from build123d import *

# Parameters (mm, degrees)
BOSS_EXTRUDE1_DEPTH     = 35
CUT_EXTRUDE1_DEPTH      = 165.23458831805192
CUT_EXTRUDE1_DEPTH_BACK = 165.23458831805192
CUT_EXTRUDE2_START      = 35
CUT_EXTRUDE2_DEPTH      = 10.61
SKETCH5_R               = 1.600000000000005
SKETCH5_R_2             = 1.6000000000000056
CUT_EXTRUDE3_DEPTH      = 165.23458831805192
SKETCH5_3_R             = 3.0000000000000004
SKETCH5_3_R_2           = 3.0000000000000013
CUT_EXTRUDE4_DEPTH      = 21
SKETCH8_R               = 1.600000000000005
SKETCH8_R_2             = 1.6000000000000056
CUT_EXTRUDE5_DEPTH      = 165.23458831805192
SKETCH8_3_R             = 3.000000000000008
CUT_EXTRUDE6_DEPTH      = 25
CUT_EXTRUDE7_REACH      = 166.235
SKETCH7_R               = 4.1
SKETCH7_R_2             = 4.099999999999986
SKETCH7_3_R             = 11
SKETCH7_3_R_2           = 10.999999999999993
CUT_EXTRUDE8_DEPTH      = 7.1
CUT_EXTRUDE9_DEPTH      = 21
CUT_EXTRUDE11_START     = 24.39
SKETCH11_R              = 11.6
CUT_EXTRUDE11_DEPTH     = 189.6245883180519
FILLET3_R               = 9
FILLET4_R               = 9


with BuildPart() as part:
    # Sketch1 → Boss-Extrude1 (new body)
    with BuildSketch(Plane(origin=(0, 0, 0), x_dir=(0, 0, -1), z_dir=(1, 0, 0))):
        with BuildLine():
            ThreePointArc((-3.4331525583588727, 27.788729073331762), (-20.97770568525129, 18.545507924642443), (-28, 3.43e-15))
            Line((-28, 0), (28, 0))
            ThreePointArc((28, 0), (18.545507924642447, 20.977705685251287), (-3.4331525583588727, 27.788729073331762))
        make_face()
        with BuildLine():
            Line((28, 0), (-28, 0))
            ThreePointArc((-28, 3.43e-15), (-20.977705685251298, -18.545507924642436), (-3.433152558358892, -27.78872907333176))
            ThreePointArc((-3.433152558358892, -27.78872907333176), (18.545507924642436, -20.977705685251298), (28, -6.86e-15))
        make_face()
        with BuildLine():
            ThreePointArc((-126.56684744164114, 27.788729073331766), (-109.02229431474872, 18.54550792464245), (-102, 0))
            Line((-102, 0), (-28, 0))
            ThreePointArc((-28, 3.43e-15), (-20.97770568525129, 18.545507924642443), (-3.4331525583588727, 27.788729073331762))
            ThreePointArc((-3.433152558358863, 27.788729073331695), (-65, 23.999999999999602), (-126.56684744164116, 27.788729073331638))
        make_face()
        with BuildLine():
            Line((-28, 0), (-102, 0))
            ThreePointArc((-102, -6.86e-15), (-109.0222943147487, -18.545507924642447), (-126.56684744164114, -27.788729073331766))
            ThreePointArc((-126.56684744164116, -27.788729073331638), (-65, -23.999999999999602), (-3.433152558358863, -27.788729073331695))
            ThreePointArc((-3.433152558358892, -27.78872907333176), (-20.977705685251298, -18.545507924642436), (-28, 3.43e-15))
        make_face()
        with BuildLine():
            ThreePointArc((-126.56684744164114, 27.788729073331766), (-148.54550792464244, 20.977705685251287), (-158, 3.43e-15))
            Line((-158, 0), (-102, 0))
            ThreePointArc((-102, 0), (-109.02229431474872, 18.54550792464245), (-126.56684744164114, 27.788729073331766))
        make_face()
        with BuildLine():
            Line((-102, 0), (-158, 0))
            ThreePointArc((-158, 3.43e-15), (-148.54550792464244, -20.97770568525128), (-126.56684744164114, -27.788729073331766))
            ThreePointArc((-126.56684744164114, -27.788729073331766), (-109.0222943147487, -18.545507924642447), (-102, -6.86e-15))
        make_face()
    extrude(amount=BOSS_EXTRUDE1_DEPTH)

    # Sketch4 → Cut-Extrude1 (cut, two sides: drawn at the far end of the back side and taken through both)
    with BuildSketch(Plane(origin=(0, 0, 0), x_dir=(1, 0, 0), z_dir=(0, 1, 0)).offset(-CUT_EXTRUDE1_DEPTH_BACK)):
        Polygon((8.999999999999998, 27.999999999999996), (61, 27.999999999999996), (61, -28.000000000000004), (9.000000000000005, -28.000000000000004), align=None)
        Polygon((60.999999999999986, -157.99999999999997), (60.99999999999993, -101.99999999999999), (8.999999999999956, -101.99999999999999), (8.99999999999997, -157.99999999999997), align=None)
    extrude(amount=CUT_EXTRUDE1_DEPTH + CUT_EXTRUDE1_DEPTH_BACK, mode=Mode.SUBTRACT)

    # Sketch6 → Cut-Extrude2 (cut)
    with BuildSketch(Plane(origin=(0, 0, 0), x_dir=(0, 0, -1), z_dir=(1, 0, 0)).offset(CUT_EXTRUDE2_START)):
        Polygon((-27.624999999999996, -21.1), (-69.825, -21.100000000000005), (-69.825, 21.099999999999994), (-27.624999999999996, 21.1), align=None)
    extrude(amount=-CUT_EXTRUDE2_DEPTH, mode=Mode.SUBTRACT)

    # Sketch5 → Cut-Extrude3 (cut, through all)
    with BuildSketch(Plane(origin=(0, 0, 0), x_dir=(0, 0, -1), z_dir=(1, 0, 0))):
        with Locations(Location((-33.225, -15.5, 0), (0, 0, 180))):
            Circle(SKETCH5_R)
        with Locations(Location((-33.225, 15.5, 0), (0, 0, 180))):
            Circle(SKETCH5_R)
        with Locations(Location((-64.22500000000001, -15.500000000000004, 0), (0, 0, 180))):
            Circle(SKETCH5_R)
        with Locations(Location((-64.22500000000001, 15.499999999999995, 0), (0, 0, 180))):
            Circle(SKETCH5_R_2)
    extrude(amount=CUT_EXTRUDE3_DEPTH, mode=Mode.SUBTRACT)

    # Sketch5<3> → Cut-Extrude4 (cut)
    with BuildSketch(Plane(origin=(0, 0, 0), x_dir=(0, 0, -1), z_dir=(1, 0, 0))):
        with Locations(Location((-33.225, -15.5, 0), (0, 0, 180))):
            Circle(SKETCH5_3_R)
        with Locations(Location((-33.225, 15.5, 0), (0, 0, 180))):
            Circle(SKETCH5_3_R)
        with Locations(Location((-64.22500000000001, -15.500000000000004, 0), (0, 0, 180))):
            Circle(SKETCH5_3_R_2)
        with Locations(Location((-64.22500000000001, 15.499999999999995, 0), (0, 0, 180))):
            Circle(SKETCH5_3_R_2)
    extrude(amount=CUT_EXTRUDE4_DEPTH, mode=Mode.SUBTRACT)

    # Sketch8 → Cut-Extrude5 (cut, through all)
    with BuildSketch(Plane(origin=(0, 0, 0), x_dir=(0, 0, -1), z_dir=(1, 0, 0))):
        with Locations((-94, -15.500000000000012)):
            Circle(SKETCH8_R)
        with Locations((-94, 15.499999999999988)):
            Circle(SKETCH8_R_2)
    extrude(amount=CUT_EXTRUDE5_DEPTH, mode=Mode.SUBTRACT)

    # Sketch8<3> → Cut-Extrude6 (cut)
    with BuildSketch(Plane(origin=(0, 0, 0), x_dir=(0, 0, -1), z_dir=(1, 0, 0))):
        with Locations((-94, -15.500000000000012)):
            Circle(SKETCH8_3_R)
        with Locations((-94, 15.499999999999988)):
            Circle(SKETCH8_3_R)
    extrude(amount=CUT_EXTRUDE6_DEPTH, mode=Mode.SUBTRACT)

    # Sketch7 → Cut-Extrude7 (cut, up to next)
    with BuildSketch(Plane(origin=(0, 0, 0), x_dir=(0, 0, -1), z_dir=(1, 0, 0)), mode=Mode.PRIVATE) as cut_extrude7_sk1:
        with Locations(Location((0, 0, 0), (0, 0, 180))):
            Circle(SKETCH7_R)
    cut_extrude7_tool1 = extrude(cut_extrude7_sk1.sketch, amount=CUT_EXTRUDE7_REACH, mode=Mode.PRIVATE) & part.part
    # Sketch7 → Cut-Extrude7 (cut, up to next)
    with BuildSketch(Plane(origin=(0, 0, 0), x_dir=(0, 0, -1), z_dir=(1, 0, 0)), mode=Mode.PRIVATE) as cut_extrude7_sk2:
        with Locations(Location((-130, 0, 0), (0, 0, 180))):
            Circle(SKETCH7_R_2)
    cut_extrude7_tool2 = extrude(cut_extrude7_sk2.sketch, amount=CUT_EXTRUDE7_REACH, mode=Mode.PRIVATE) & part.part
    add(cut_extrude7_tool1.solids().sort_by_distance((0, 0, 0))[0], mode=Mode.SUBTRACT)
    add(cut_extrude7_tool2.solids().sort_by_distance((0, 0, 130))[0], mode=Mode.SUBTRACT)

    # Sketch7<3> → Cut-Extrude8 (cut)
    with BuildSketch(Plane(origin=(0, 0, 0), x_dir=(0, 0, -1), z_dir=(1, 0, 0))):
        Circle(SKETCH7_3_R)
        with Locations((-130, 0)):
            Circle(SKETCH7_3_R_2)
    extrude(amount=CUT_EXTRUDE8_DEPTH, mode=Mode.SUBTRACT)

    # Sketch9 → Cut-Extrude9 (cut)
    with BuildSketch(Plane(origin=(0, 0, 0), x_dir=(0, 0, -1), z_dir=(1, 0, 0))):
        with BuildLine():
            Line((-52.942405411719506, -6.7980505730098315), (-34.806527029394815, -18.04926896487869))
            ThreePointArc((-34.80652702939481, -18.049268964878678), (-34.68366701337481, -12.878494603459266), (-30.22500000000001, -15.5))
            Line((-30.225000000000005, -15.5), (-30.225000000000005, 15.5))
            ThreePointArc((-30.225, 15.5), (-34.68366701337481, 12.878494603459261), (-34.806527029394815, 18.04926896487868))
            Line((-34.806527029394815, 18.04926896487869), (-52.942405411719506, 6.7980505730098315))
            ThreePointArc((-52.9424054117195, 6.7980505730098155), (-56.725, 9.8e-16), (-52.9424054117195, -6.798050573009815))
        make_face()
    extrude(amount=CUT_EXTRUDE9_DEPTH, mode=Mode.SUBTRACT)

    # Sketch11 → Cut-Extrude11 (cut, through all)
    with BuildSketch(Plane(origin=(0, 0, 0), x_dir=(0, 0, -1), z_dir=(1, 0, 0)).offset(CUT_EXTRUDE11_START)):
        with Locations(Location((-48.725, 0, 0), (0, 0, 75.417643506))):
            Circle(SKETCH11_R)
    extrude(amount=-CUT_EXTRUDE11_DEPTH, mode=Mode.SUBTRACT)

    # Fillet3
    # the kernel refuses this fillet: 9 mm, written as the material it takes off along each edge
    with BuildSketch(Plane(origin=(0, -7.11e-15, 130), x_dir=(0, 0.9924546097618487, -0.12261259136995861), z_dir=(0, -0.12261259136995861, -0.9924546097618487))) as fillet3_piece_1:
        with BuildLine():
            CenterArc((28 - FILLET3_R, FILLET3_R), FILLET3_R, 270, 89.99999999999999)
            Line((28, FILLET3_R), (28, 0))
            Line((28, 0), (28 - FILLET3_R, 0))
        make_face()
    revolve(axis=Axis((0, -7.11e-15, 130), (1, 0, 0)), revolution_arc=194.0858135076888, mode=Mode.SUBTRACT)
    with BuildSketch(Plane(origin=(0, -526.1249999999588, 65.00000000000026), x_dir=(0, 0.9924546097618475, 0.12261259136996942), z_dir=(0, -0.12261259136996942, 0.9924546097618475))) as fillet3_piece_2:
        with BuildLine():
            CenterArc((502.1249999999593 + FILLET3_R, -FILLET3_R), FILLET3_R, 90, 90)
            Line((502.1249999999593 + FILLET3_R, 1.78e-15), (502.1249999999593, 0))
            Line((502.1249999999593, 0), (502.1249999999593, -FILLET3_R))
        make_face()
    revolve(axis=Axis((0, -526.1249999999588, 65.00000000000026), (-1, 0, 0)), revolution_arc=14.085813507690109, mode=Mode.SUBTRACT)
    with BuildSketch(Plane(origin=(0, 1.78e-15, -1.78e-15), x_dir=(0, -0.9924546097618486, 0.12261259136995943), z_dir=(0, 0.12261259136995943, 0.9924546097618486))) as fillet3_piece_3:
        with BuildLine():
            CenterArc((27.999999999999993 - FILLET3_R, FILLET3_R), FILLET3_R, 270, 89.99999999999999)
            Line((27.999999999999993, FILLET3_R), (27.999999999999993, 0))
            Line((27.999999999999993, 0), (27.999999999999993 - FILLET3_R, 0))
        make_face()
    revolve(axis=Axis((0, 1.78e-15, -1.78e-15), (1, 0, 0)), revolution_arc=194.0858135076889, mode=Mode.SUBTRACT)
    with BuildSketch(Plane(origin=(0, 526.1249999999663, 65.00000000000024), x_dir=(0, -0.9924546097618476, -0.12261259136996856), z_dir=(0, 0.12261259136996856, -0.9924546097618476))) as fillet3_piece_4:
        with BuildLine():
            CenterArc((502.1249999999667 + FILLET3_R, -FILLET3_R), FILLET3_R, 90, 90)
            Line((502.1249999999667 + FILLET3_R, 1.78e-15), (502.1249999999667, 0))
            Line((502.1249999999667, 0), (502.1249999999667, -FILLET3_R))
        make_face()
    revolve(axis=Axis((0, 526.1249999999663, 65.00000000000024), (-1, 0, 0)), revolution_arc=14.085813507689899, mode=Mode.SUBTRACT)

    # Fillet4
    fillet4_edges = [part.edges().sort_by_distance(p)[0] for p in [
        (22.000000000000004, -25.365061880944552, 28),
        (21.99999999999998, -25.365061880944495, 101.99999999999999),
        (21.99999999999998, 25.365061880944552, 101.99999999999999),
        (22.000000000000004, 25.36506188094461, 28),
    ]]
    fillet(fillet4_edges, radius=FILLET4_R)


solid = part.part
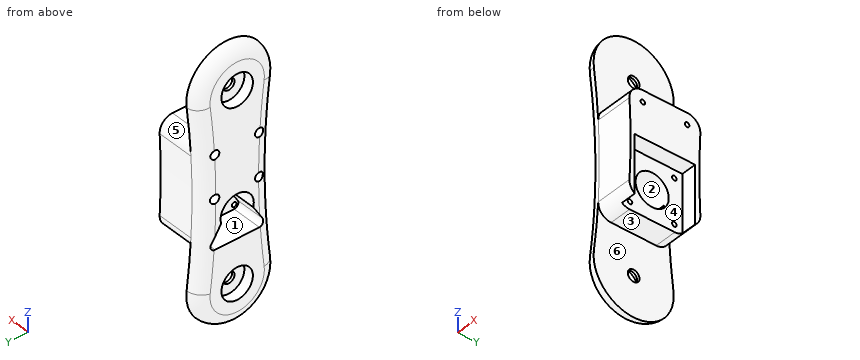
Can you work these out from the model? Positions are in its coordinate system, mm. Face numbers are marked on the shaded views. A direction names the side the tool comes from. Round coordinates to 2 decimals unless told otherwise and drop trailing zeros. Order: outer loops, then holes, each group sorted by start corner. A loop starts at its lowest first (then second) coordinate and runs counter-clockwise, first axis right, second up. Notation, with made-up numbers: M 35,74 L 74,74 A22 cw 74,106 Z; hole C 33.5,26 d11. An arc over 180 degrees is marked long. Use a Markdown table: item, result.
1) Imagine slicing it at C-C (x = 14.5). List the corners of the cut face in (y, z) for me (3 decimals), then the cut area to 3 significant figures.
Geometry says:
| item | result |
|---|---|
| outline | M -24.754,37.493 A9 ccw -15.768,28 L 15.768,28 A9 ccw 24.754,37.493 A502.125 cw 24.754,92.507 A9 ccw 15.768,102 L -15.768,102 A9 ccw -24.754,92.507 A502.125 cw Z; hole C -15.5,64.225 d6; hole C -15.5,94 d6; hole M -18.049,34.807 A3 ccw -15.5,30.225 L 15.5,30.225 A3 ccw 18.049,34.807 L 11.226,45.804 A11.6 ccw long -11.226,45.804 Z; hole C 15.5,64.225 d6; hole C 15.5,94 d6 |
| area | 2,660 mm² |
2) Imagine slicing it at D-D (x = 3). List the corners of the cut face in (y, z) for me (3 decimals), then the cut area to 3 significant figures.
Geometry says:
| item | result |
|---|---|
| outline | M -25.514,3.152 A25.708 ccw long 25.514,3.152 A504.417 cw 25.514,126.848 A25.708 ccw long -25.514,126.848 A504.417 cw Z; hole C -15.5,64.225 d6; hole C -15.5,94 d6; hole M -18.049,34.807 A3 ccw -15.5,30.225 L 15.5,30.225 A3 ccw 18.049,34.807 L 11.226,45.804 A11.6 ccw long -11.226,45.804 Z; hole C 0,0 d22; hole C 0,130 d22; hole C 15.5,64.225 d6; hole C 15.5,94 d6 |
| area | 6,440 mm² |
3) If I drill on line 1 along Z through (x, y) = (15.25, -15.5) (3 decimals); line 2 along Y through (x, z) = (8.35, 130); line 3 along Z through (x, y) = (3, -17.5), over which ranges is the centre line in solid material (lowest first)?
Geometry says:
| item | result |
|---|---|
| line 1 | z = 28 to 30.225, 38.916 to 61.225, 67.225 to 91, 97 to 102 |
| line 2 | y = -27.98 to -4.1, 4.1 to 27.98 |
| line 3 | z = -18.83 to 30.99, 35.69 to 61.99, 66.46 to 91.76, 96.24 to 148.83 |
4) Imagine slicing it at A-A (z = 0). List the corners of the cut face in (x, y) for me, then the cut area to 3 significant figures.
Geometry says:
| item | result |
|---|---|
| outline | M 0,-19 A9 ccw 9,-28 L 9,-4.1 L 7.1,-4.1 L 7.1,-11 L 0,-11 Z; M 0,11 L 7.1,11 L 7.1,4.1 L 9,4.1 L 9,28 A9 ccw 0,19 Z |
| area | 297 mm² |
5) On a 3-axis mill with a long thin cutter (end or side, diameter ignored), from which of +Z, -Z, +X, -X, +Y, -Y can I reach the whole of each face in a straight line? I mean the marked faces 1, 2 and 3. Say none if no direction works.
Geometry says:
| item | result |
|---|---|
| face 1 | -X |
| face 2 | +X, -X |
| face 3 | -Z, +X, +Y, -Y |
6) I'm going to push flat-ended pins straight in: P1, Ø6, axis at x = 20.5, y = 7, coming from the -Z side; P2, Ø13, axis at y = 0, z = 0, coming from the -X side; P3, Ø20, axis at y = 0, z = 130, coming from the +X side. Where does each tip first touch, or does it pass through?
Geometry says:
| item | result |
|---|---|
| P1 | stops at z = 28 |
| P2 | stops at x = 7.1 |
| P3 | stops at x = 9 |
7) If we mould it in two halves opening along Y, with no side actions, what happens to the marked faces 4, 5 and 6? For each: +Y half, -Y half, draft (parallel to the pull), parting line (faces both ways), or undercut.
Geometry says:
| item | result |
|---|---|
| face 4 | undercut |
| face 5 | +Y half |
| face 6 | draft |
8) Imagine slicing it at B-B (x = 29). List the corners of the cut face in (y, z) for me (3 decimals).
Geometry says:
| item | result |
|---|---|
| outline | M -24.754,37.493 A9 ccw -21.1,29.75 L -21.1,69.825 L 21.1,69.825 L 21.1,29.75 A9 ccw 24.754,37.493 A502.125 cw 24.754,92.507 A9 ccw 15.768,102 L -15.768,102 A9 ccw -24.754,92.507 A502.125 cw Z; hole C -15.5,94 d3.2; hole C 15.5,94 d3.2 |
